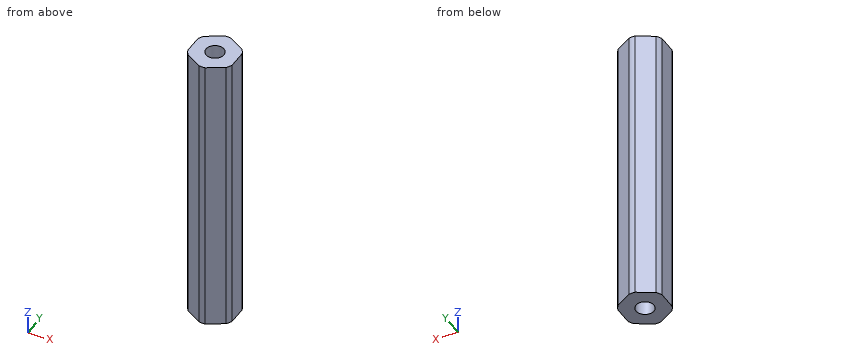
Autodesk Inventor part; units mm, degrees
ref_plane "YZ Plane" through (0, 0, 0) normal (1, 0, 0) x (0, 1, 0)
ref_plane "XZ Plane" through (0, 0, 0) normal (0, 1, 0) x (-1, 0, 0)
ref_plane "XY Plane" through (0, 0, 0) normal (0, 0, 1) x (1, 0, 0)
sketch "Sketch1" plane through (0, 0, 0) normal (0, 0, 1) x (1, 0, 0)
  line L0 (-6.35, -3.6662) -> (-6.35, 3.6662)
  line L1 (-6.35, 3.6662) -> (0, 7.3323)
  line L2 (0, 7.3323) -> (6.35, 3.6662)
  line L3 (6.35, 3.6662) -> (6.35, -3.6662)
  line L4 (6.35, -3.6662) -> (0, -7.3323)
  line L5 (0, -7.3323) -> (-6.35, -3.6662)
  point P0 (0, 0)
  point P1 (0, 0)
  dimension "Size" = 12.7
extrude "Extrusion1" add sketch "Sketch1" along normal mid plane 82.55
sketch "Sketch3" plane through (0, 0, 41.275) normal (0, 0, 1) x (1, 0, 0)
  line L0 (-6.35, 3.6662) -> (0, 7.3323) construction
  line L1 (0, 7.3323) -> (6.35, 3.6662) construction
  line L2 (6.35, 3.6662) -> (6.35, -3.6662) construction
  line L3 (6.35, -3.6662) -> (0, -7.3323) construction
  line L4 (0, -7.3323) -> (-6.35, -3.6662) construction
  line L5 (-6.35, -3.6662) -> (-6.35, 3.6662) construction
  point P0 (0, 0)
hole "Hole1" at (0, 0, 41.275) direction (0, 0, -1) diameter 5.1054 end through all
sketch "Sketch4" plane through (0, 0, 41.275) normal (0, 0, 1) x (1, 0, 0)
  circle A0 centre (0, 0) radius 2.5527 construction
  line L0 (-6.35, 3.6662) -> (0, 7.3323) construction
  line L1 (0, 7.3323) -> (6.35, 3.6662) construction
  line L2 (6.35, 3.6662) -> (6.35, -3.6662) construction
  line L3 (6.35, -3.6662) -> (0, -7.3323) construction
  line L4 (0, -7.3323) -> (-6.35, -3.6662) construction
  line L5 (-6.35, -3.6662) -> (-6.35, 3.6662) construction
  circle A1 centre (0, 0) radius 6.8771
  circle A2 centre (0, 0) radius 8.89
  dimension "thunder" = 13.7541
  dimension "d16" = 17.78
extrude "Extrusion3" cut sketch "Sketch4" against normal through all
equation "\"bearing\" = 25.4"
properties part number "GP10-006" material "Aluminum 6061"
Part model, mm, in its own coordinate system. Give positions to 0.01 mm unless a question says otherwise; leave off trailing zeros. Order: outer loops, then holes, each group sorted by start corner. A loop starts at its lowest first (then second) coordinate and runs counter-clockwise, first axis right, second up. Notation, with made-up numbers: (83, 13) - (107, 13) arc R19 ccw to (107, 48) - close; hole circle Ø3 at (85.25, 83). An arc over 180 degrees is marked (long way). One line per question, with ' | ' between items.
1. Band-saw the part on B-B on x = 0. List the corners of the cut face in (y, z) (3 decimals).
Filled in:
outline: (-6.877, -41.275) - (-2.553, -41.275) - (-2.553, 41.275) - (-6.877, 41.275) - close; (2.553, -41.275) - (6.877, -41.275) - (6.877, 41.275) - (2.553, 41.275) - close
2. Drop flat-ended pins along their axis: P1, Ø1.5, axis at y = -3, z = -4, coming from the -X side; P2, Ø3, axis at y = 5, z = 4, coming from the +X side; P3, Ø4.5, axis at x = 0, y = 0, coming from the +Z side. Give the stop position or say it passes through.
Filled in:
P1: x = -6.35 | P2: x = 5.92 | P3: through
3. Band-saw the part on D-D on y = 5. List the corners of the cut face in (x, z) (3 decimals).
Filled in:
outline: (-4.04, -41.275) - (4.04, -41.275) - (4.04, 41.275) - (-4.04, 41.275) - close
4. Band-saw the part on A-A on y = 0. List the corners of the cut face in (x, z) (3 decimals).
Filled in:
outline: (-6.35, -41.275) - (-2.553, -41.275) - (-2.553, 41.275) - (-6.35, 41.275) - close; (2.553, -41.275) - (6.35, -41.275) - (6.35, 41.275) - (2.553, 41.275) - close
5. Band-saw the part on C-C on z = 32. List the corners of the cut face in (x, y), then the cut area to 3 significant figures.
Filled in:
outline: (-6.35, -2.64) arc R6.88 ccw to (-5.46, -4.18) - (-0.89, -6.82) arc R6.88 ccw to (0.89, -6.82) - (5.46, -4.18) arc R6.88 ccw to (6.35, -2.64) - (6.35, 2.64) arc R6.88 ccw to (5.46, 4.18) - (0.89, 6.82) arc R6.88 ccw to (-0.89, 6.82) - (-5.46, 4.18) arc R6.88 ccw to (-6.35, 2.64) - close; hole circle Ø5.11 at (0, 0) | area: 117 mm²
6. Drill centre lines: probe 1 along X at (y, z) = (0, -14.5); probe 2 along Y at (x, z) = (2, -23.5); probe 3 along Y at (x, z) = (0.75, -13.5). Where is each one in solid material? Low to high.
Filled in:
probe 1: -6.35 to -2.55, 2.55 to 6.35 | probe 2: -6.18 to -1.59, 1.59 to 6.18 | probe 3: -6.84 to -2.44, 2.44 to 6.84
